Can you work these out from the model? Positions are in its coordinate system, mm. A direction names the side the tool comes from. Coordinates: 2 decimals unless noted, no trailing zeros. Loops run counter-clockwise (first coordinate to the right, second up) from the corner with the lowest first, then second, coordinate; pieces in that order, holes last.
```python
from build123d import *

# Parameters (mm, degrees)
SKETCH_1_W             = 6
SKETCH_1_H             = 50
SKETCH_1_W_2           = 3
HOLE_WIZARD_M4_1_D     = 3.3
HOLE_WIZARD_M4_1_DEPTH = 10
HOLE_WIZARD_M4_1_TIP   = 0.991420021
EXTRUDE_1_DEPTH        = 50
SKETCH_7_R             = 29
SKETCH_7_R_2           = 26
EXTRUDE_3_DEPTH        = 6
CHAMFER_1_SIZE         = 0.5
FILLET_1_R             = 5


with BuildPart() as part:
    # 草图1 → 旋转1 (revolve)
    with BuildSketch(Plane.XY, mode=Mode.PRIVATE) as revolve_1_sk:
        with Locations((27.5, 25)):
            Rectangle(SKETCH_1_W, SKETCH_1_H)
        with Locations((68.5, 25)):
            Rectangle(SKETCH_1_W_2, SKETCH_1_H)
    revolve(revolve_1_sk.sketch.rotate(Axis((0, 82.659451531, 0), (0, -1, 0)), 90), axis=Axis((0, 82.659451531, 0), (0, -1, 0)))

    # M4 螺纹孔1
    with Locations(Plane(origin=(0, 0, 0), x_dir=(-1, 0, 0), z_dir=(0, -1, 0))):
        with Locations((0, 27.5), (19.445436483, -19.445436483), (27.5, 0), (19.445436483, 19.445436483), (0, -27.5), (-19.445436483, -19.445436483), (-27.5, 0), (-19.445436483, 19.445436483)):
            Hole(HOLE_WIZARD_M4_1_D / 2, depth=HOLE_WIZARD_M4_1_DEPTH)
            with Locations((0, 0, -(HOLE_WIZARD_M4_1_DEPTH + HOLE_WIZARD_M4_1_TIP / 2))):  # 118° drill point
                Cone(0, HOLE_WIZARD_M4_1_D / 2, HOLE_WIZARD_M4_1_TIP, mode=Mode.SUBTRACT)

    # 草图5 → 凸台-拉伸1 (add)
    with BuildSketch(Plane(origin=(0, 50, 0), x_dir=(1, 0, 0), z_dir=(0, 1, 0))):
        with BuildLine():
            Line((1, -66.992536898), (2, -30.434355587))
            ThreePointArc((2, -30.434355587), (0, -30.5), (-2, -30.434355587))
            Line((-2, -30.434355587), (-1, -66.992536898))
            ThreePointArc((-1, -66.992536898), (0, -67), (1, -66.992536898))
        make_face()
        with BuildLine():
            ThreePointArc((-28.326758212, -11.306846122), (-29.007223747, -9.425018328), (-29.562826189, -7.502620057))
            Line((-29.562826189, -7.502620057), (-64.022705754, -19.750775881))
            ThreePointArc((-64.022705754, -19.750775881), (-63.720786592, -20.704138623), (-63.404671765, -21.652888914))
            Line((-63.404671765, -21.652888914), (-28.326758212, -11.306846122))
        make_face()
        with BuildLine():
            ThreePointArc((-19.506899366, 23.446340378), (-17.927450195, 24.675018328), (-16.270831388, 25.797481387))
            Line((-16.270831388, 25.797481387), (-38.568208208, 54.785886099))
            ThreePointArc((-38.568208208, 54.785886099), (-39.381611904, 54.204138623), (-40.186242197, 53.610315594))
            Line((-40.186242197, 53.610315594), (-19.506899366, 23.446340378))
        make_face()
        with BuildLine():
            ThreePointArc((16.270831388, 25.797481387), (17.927450195, 24.675018328), (19.506899366, 23.446340378))
            Line((19.506899366, 23.446340378), (40.186242197, 53.610315594))
            ThreePointArc((40.186242197, 53.610315594), (39.381611904, 54.204138623), (38.568208208, 54.785886099))
            Line((38.568208208, 54.785886099), (16.270831388, 25.797481387))
        make_face()
        with BuildLine():
            ThreePointArc((29.562826189, -7.502620057), (29.007223747, -9.425018328), (28.326758212, -11.306846122))
            Line((28.326758212, -11.306846122), (63.404671765, -21.652888914))
            ThreePointArc((63.404671765, -21.652888914), (63.720786592, -20.704138623), (64.022705754, -19.750775881))
            Line((64.022705754, -19.750775881), (29.562826189, -7.502620057))
        make_face()
    extrude(amount=-EXTRUDE_1_DEPTH)

    # 草图7 → 凸台-拉伸3 (add)
    with BuildSketch(Plane(origin=(0, 50, 0), x_dir=(1, 0, 0), z_dir=(0, 1, 0))):
        with Locations(Location((0, 0, 0), (0, 0, 270))):
            Circle(SKETCH_7_R)
        with Locations(Location((0, 0, 0), (0, 0, 270))):
            Circle(SKETCH_7_R_2, mode=Mode.SUBTRACT)
    extrude(amount=EXTRUDE_3_DEPTH)

    # 倒角1
    chamfer_1_edges = [part.edges().sort_by_distance(p)[0] for p in [
        (0, 56, -26),
        (0, 0, -24.5),
    ]]
    chamfer(chamfer_1_edges, length=CHAMFER_1_SIZE)

    # 圆角1
    fillet_1_edges = [part.edges().sort_by_distance(p)[0] for p in [
        (-2, 25, 30.434355587),
        (2, 25, 30.434355587),
        (1, 25, 66.992536898),
        (-1, 25, 66.992536898),
        (-29.562826189, 25, 7.502620057),
        (-28.326758212, 25, 11.306846122),
        (-63.404671765, 25, 21.652888914),
        (-64.022705754, 25, 19.750775881),
        (-16.270831388, 25, -25.797481387),
        (-19.506899366, 25, -23.446340378),
        (-40.186242197, 25, -53.610315594),
        (-38.568208208, 25, -54.785886099),
        (19.506899366, 25, -23.446340378),
        (16.270831388, 25, -25.797481387),
        (38.568208208, 25, -54.785886099),
        (40.186242197, 25, -53.610315594),
        (28.326758212, 25, 11.306846122),
        (29.562826189, 25, 7.502620057),
        (64.022705754, 25, 19.750775881),
        (63.404671765, 25, 21.652888914),
    ]]
    fillet(fillet_1_edges, radius=FILLET_1_R)


solid = part.part
```
Item 1: We'd pull the mould along Z, two halves only. Please class faces 1 (the face through (-21.1, 50, 20.4)), 2 (the face through (19.48, 10.82, -19.73)): +Z half, -Z half, draft (parallel to the pull), parting line (faces both ways), or undercut.
Results are:
face 1: draft
face 2: undercut
Item 2: I'm going to push flat-ended pins straight in: P1, Ø1.5, axis at y = 12, z = -12.5, coming from the -X side; P2, Ø2, axis at x = 27.5, z = 0, coming from the -Y side; P3, Ø4, axis at y = 47, z = 28.5, coming from the -X side; P4, Ø12, axis at x = 1.5, z = -14.5, coming from the +Y side. Where does each tip first touch, or does it pass through?
Results are:
P1: stops at x = -69.01
P2: stops at y = 10.39
P3: stops at x = -64.79
P4: passes through
Item 3: Suppose I cut it at B-B, the plane z = -15. Count the separate pieces of the cut face and the enclosed holes in it, plus the area to 3 significant figures.
Results are:
separate pieces: 4
enclosed holes: 0
area: 1,070 mm2
Item 4: I need wall thicknesses on line 1 along X through (y, z) = (26, 0); line 2 along X through (y, z) = (34, -37.5); line 3 along X through (y, z) = (52.9, 0). Which ranges of each line are inside material? Lowest first, please.
Results are:
line 1: x = -70 to -67, -30.5 to -24.5, 24.5 to 30.5, 67 to 70
line 2: x = -59.11 to -55.52, -29.14 to -25.27, 25.27 to 29.14, 55.52 to 59.11
line 3: x = -29 to -26, 26 to 29
Item 5: On a 3-axis mill with a long thin cutter (end or side, diameter ignored), from which of +Z, -Z, +X, -X, +Y, -Y can I reach the whole of each face in a straight line? I mean faces 3 (the face through (-29.62, 25.35, -38.2)), 4 (the face through (25.85, 5.07, -0.07)). Say none if no direction works.
Results are:
face 3: +Y, -Y
face 4: -Y
Item 6: Suppose I cut it at A-A, the plane z = 44.5. Please give me the cut outline in (x, y), plus the area to 3 significant figures.
Results are:
outline: (-54.03, 0) - (-50.09, 0) - (-50.09, 50) - (-54.03, 50) - close; (-1.62, 0) - (1.62, 0) - (1.62, 50) - (-1.62, 50) - close; (50.09, 0) - (54.03, 0) - (54.03, 50) - (50.09, 50) - close
area: 556 mm2
